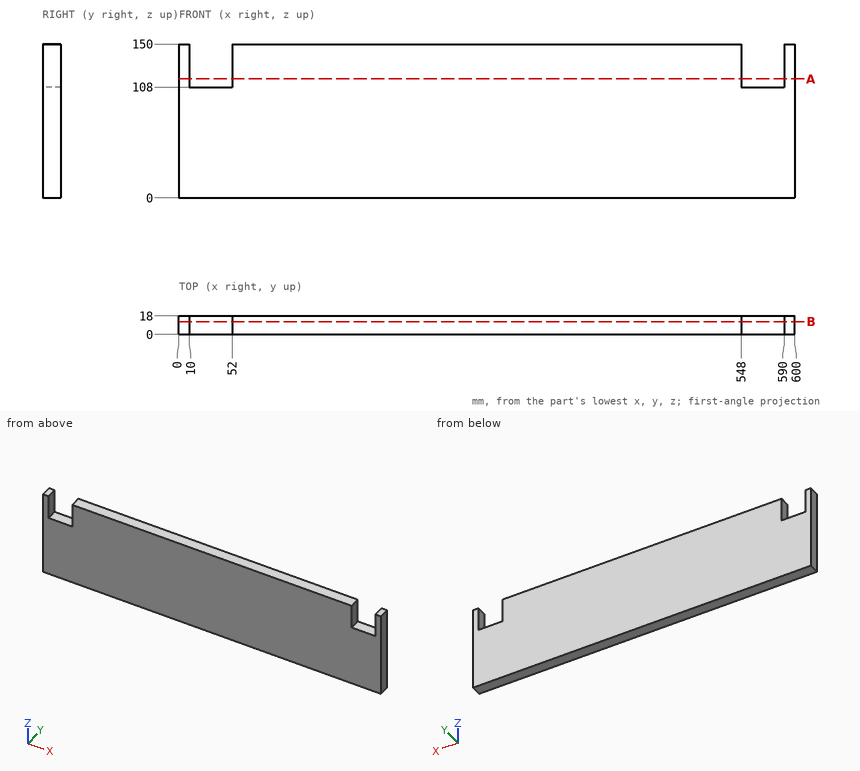
The drawing under review shows one solid part. Ordinate dimensions are in mm from its lowest x, y, z. Coordinates: 2 decimals unless noted, no trailing zeros. Write each loop counter-clockwise with the first axis right and the second up, starting at its lowest first coordinate (ties: lowest second). Pieces come first, ordered by that corner, then holes. Notation, with made-up numbers: (-20.5, 63) - (-8.5, 63) arc R27 ccw to (-8.5, 88) - close; hole circle Ø8 at (60.25, 64.25). An arc over 180 degrees is marked (long way). Put each result on its own line as item: value.
1. Add section B-B, the plane y = 12.5. Give the boundary of the cut face in (x, z), then the cut area to 3 significant figures.
Values found:
outline: (0, 0) - (600, 0) - (600, 150) - (590, 150) - (590, 108) - (548, 108) - (548, 150) - (52, 150) - (52, 108) - (10, 108) - (10, 150) - (0, 150) - close
area: 86,500 mm²
2. Wall thickness on probe 1 along X at (y, z) = (8.5, 121.5); probe 2 along Z at (x, y) = (572.5, 4.75): over which ranges is each line inside the solid? List them lowest first.
Values found:
probe 1: 0 to 10, 52 to 548, 590 to 600
probe 2: 0 to 108
3. Add section A-A, the plane z = 116. Give the boundary of the cut face in (x, y).
Values found:
outline: (0, 0) - (10, 0) - (10, 18) - (0, 18) - close; (52, 0) - (548, 0) - (548, 18) - (52, 18) - close; (590, 0) - (600, 0) - (600, 18) - (590, 18) - close
